from build123d import *

# Parameters (mm, degrees)
SKETCH1_R               = 32
BOSS_EXTRUDE1_DEPTH     = 0.999998
SKETCH8_R               = 30
SKETCH8_R_2             = 28.5
BOSS_EXTRUDE4_DEPTH     = 5
SKETCH9_R               = 5.207
BOSS_EXTRUDE5_DEPTH     = 5
CUT_EXTRUDE1_DEPTH      = 1
CUT_EXTRUDE1_DEPTH_BACK = 7.999996
SKETCH10_R              = 2.8067
CUT_EXTRUDE2_DEPTH      = 4.7
CUT_EXTRUDE2_TAPER      = 8


with BuildPart() as part:
    # Sketch1 → Boss-Extrude1 (new body, symmetric)
    with BuildSketch(Plane.XY):
        Circle(SKETCH1_R)
    extrude(amount=BOSS_EXTRUDE1_DEPTH, both=True)

    # Sketch8 → Boss-Extrude4 (add)
    with BuildSketch(Plane.XY.offset(0.999998)):
        Circle(SKETCH8_R)
        Circle(SKETCH8_R_2, mode=Mode.SUBTRACT)
    extrude(amount=BOSS_EXTRUDE4_DEPTH)

    # Sketch9 → Boss-Extrude5 (add)
    with BuildSketch(Plane.XY.offset(0.999998)):
        with Locations((0, 17.4498)):
            Circle(SKETCH9_R)
        with Locations((0, -17.4498)):
            Circle(SKETCH9_R)
    extrude(amount=BOSS_EXTRUDE5_DEPTH)

    # Sketch7 → Cut-Extrude1 (cut, two sides)
    with BuildSketch(Plane(origin=(0, 0, -0.999998), x_dir=(-1, 0, 0), z_dir=(0, 0, -1))) as cut_extrude1_sk:
        with BuildLine():
            Line((14.45, 1.8542), (14.45, -7.0358))
            ThreePointArc((14.45, -7.0358), (12.7, -8.7858), (10.95, -7.0358))
            Line((10.95, -7.0358), (10.95, 1.8542))
            ThreePointArc((10.95, 1.8542), (12.7, 3.6042), (14.45, 1.8542))
        make_face()
    extrude(amount=CUT_EXTRUDE1_DEPTH, mode=Mode.SUBTRACT)
    extrude(cut_extrude1_sk.sketch, amount=-CUT_EXTRUDE1_DEPTH_BACK, mode=Mode.SUBTRACT)

    # Sketch10 → Cut-Extrude2 (cut)
    with BuildSketch(Plane.XY.offset(5.999998)):
        with Locations((0, 17.4498)):
            Circle(SKETCH10_R)
        with Locations((0, -17.4498)):
            Circle(SKETCH10_R)
    extrude(amount=-CUT_EXTRUDE2_DEPTH, taper=CUT_EXTRUDE2_TAPER, mode=Mode.SUBTRACT)


solid = part.part
The listing builds one solid part. Answer for the finished solid, in the listing's coordinates (mm). A direction names the side the tool comes from. Coordinates: 2 decimals unless noted, no trailing zeros. Write each loop counter-clockwise with the first axis right and the second up, starting at its lowest first coordinate (ties: lowest second). Pieces come first, ordered by that corner, then holes. Notation, with made-up numbers: (75.5, 71) - (125.5, 71) arc R4 cw to (125.5, 76) - close; hole circle Ø4 at (11, 18). An arc over 180 degrees is marked (long way). Put each result on its own line as item: value.
1. Flat-ended cylindrical pins translate along their axes: pin 1 Ø1 at (x, z) = (-13.5, 3) entering from -Y; pin 2 Ø1 at (x, z) = (-13, 1) entering from +Y; pin 3 Ø1 at (y, z) = (-4.5, -0.5) entering from +X. Find the tip coordinate at first contact, or state that the pin passes through.
Answer sheet:
pin 1: stops at y = -27.04
pin 2: stops at y = 29.46
pin 3: stops at x = 31.75
2. The part is cut by section C-C on z = 2.5. Give the vertices of the cut face in (x, y).
Answer sheet:
outline: circle Ø60 at (0, 0); circle Ø10.41 at (0, -17.45); circle Ø10.41 at (0, 17.45); hole circle Ø57 at (0, 0); hole circle Ø4.63 at (0, -17.45); hole circle Ø4.63 at (0, 17.45)
3. Find the intervals of material crossed by line 1 along Y through (x, z) = (0, 2.95); line 2 along X through (y, z) = (-21.5, 3.5); line 3 along Y through (x, z) = (0, 3.85), in increasing order. Write a range as from..to.
Answer sheet:
line 1: y = -30..-28.5, -22.66..-19.83, -15.07..-12.24, 12.24..15.07, 19.83..22.66, 28.5..30
line 2: x = -20.92..-18.71, -3.27..3.27, 18.71..20.92
line 3: y = -30..-28.5, -22.66..-19.95, -14.95..-12.24, 12.24..14.95, 19.95..22.66, 28.5..30
4. The part is cut by section D-D on x = -12.7. Give the vertices of the cut face in (y, z), plus the area to 3 significant figures.
Answer sheet:
outline: (-29.37, -1) - (-8.79, -1) - (-8.79, 1) - (-25.51, 1) - (-25.51, 6) - (-27.18, 6) - (-27.18, 1) - (-29.37, 1) - close; (3.6, -1) - (29.37, -1) - (29.37, 1) - (27.18, 1) - (27.18, 6) - (25.51, 6) - (25.51, 1) - (3.6, 1) - close
area: 109 mm^2
5. The part is cut by section A-A on y = 0. Give the vertices of the cut face in (x, z), plus the area to 3 significant figures.
Answer sheet:
outline: (-32, -1) - (-14.45, -1) - (-14.45, 1) - (-28.5, 1) - (-28.5, 6) - (-30, 6) - (-30, 1) - (-32, 1) - close; (-10.95, -1) - (32, -1) - (32, 1) - (30, 1) - (30, 6) - (28.5, 6) - (28.5, 1) - (-10.95, 1) - close
area: 136 mm^2
6. A tool of negligible diameter and unlimited length cuts with its end or side. For faces 4 (the face through (11, -27, 6)), 5 (the face through (-14.45, -3, 0)), 6 (the face through (0, 0, 1)), from which of +Z, -Z, +X, -X, +Y, -Y can it reach the whole face along a straight path? Write none if from no direction.
Answer sheet:
face 4: +Z, +X, -X, +Y, -Y
face 5: +Z, -Z
face 6: +Z
7. The part is cut by section B-B on x = 0. Give the vertices of the cut face in (y, z).
Answer sheet:
outline: (-32, -1) - (32, -1) - (32, 1) - (30, 1) - (30, 6) - (28.5, 6) - (28.5, 1) - (22.66, 1) - (22.66, 6) - (20.26, 6) - (19.6, 1.3) - (15.3, 1.3) - (14.64, 6) - (12.24, 6) - (12.24, 1) - (-12.24, 1) - (-12.24, 6) - (-14.64, 6) - (-15.3, 1.3) - (-19.6, 1.3) - (-20.26, 6) - (-22.66, 6) - (-22.66, 1) - (-28.5, 1) - (-28.5, 6) - (-30, 6) - (-30, 1) - (-32, 1) - close
8. Determine the mould class of faces 1 (the face through (0, 0, -1)), 2 (the face through (26.327, -10.916, 3.465)), 3 (the face through (-29.97, 1.32, 3.46)) for opening direction X: pulls with the +X half, pulls with the -X half, needs draft (parallel to the pull), parting line crosses it, or undercut.
Answer sheet:
face 1: needs draft
face 2: undercut
face 3: parting line crosses it
